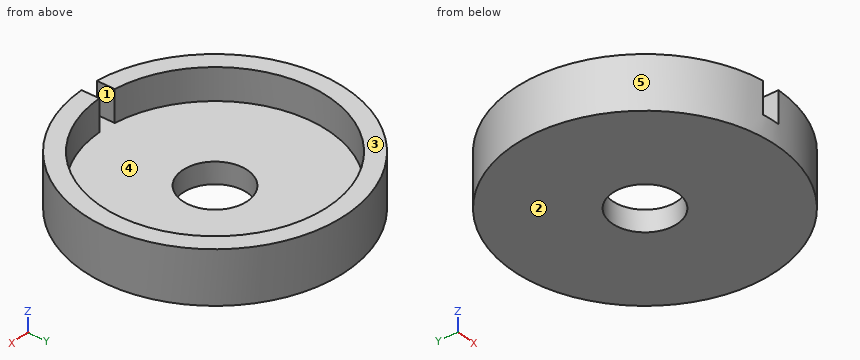
from build123d import *

# Parameters (mm, degrees)
F0_R     = 7.5
F1_DEPTH = 3
F2_R     = 6.5000001341
F3_DEPTH = 1.8
F5_DEPTH = 1.8
F6_R     = 1.85
F7_DEPTH = 2


with BuildPart() as f1:
    # F0 (on Top) → F1 (new body)
    with BuildSketch(Plane.XY):
        Circle(F0_R)
    extrude(amount=F1_DEPTH)

    # F2 (on face) → F3 (cut)
    with BuildSketch(Plane.XY.offset(3)):
        Circle(F2_R)
    extrude(amount=-F3_DEPTH, mode=Mode.SUBTRACT)

    # F4 (on face) → F5 (cut)
    with BuildSketch(Plane.XY.offset(3)):
        with BuildLine():
            Line((0, -7.5), (0, -6.5000001341))
            ThreePointArc((0, -6.5000001341), (-0.4891376474, -6.4815697254), (-0.9755014466, -6.4263830162))
            Line((-0.9755014466, -6.4263830162), (-0.9755014466, -7.4362891907))
            ThreePointArc((-0.9755014466, -7.4362891907), (-0.4887898678, -7.4840553489), (0, -7.5))
        make_face()
    extrude(amount=-F5_DEPTH, mode=Mode.SUBTRACT)

    # F6 (on face) → F7 (cut)
    with BuildSketch(Plane.XY.offset(1.2)):
        Circle(F6_R)
    extrude(amount=-F7_DEPTH, mode=Mode.SUBTRACT)


solid = f1.part
The model under review builds one solid part; all positions refer to its coordinate system, in mm. Face numbers are marked on the shaded views. A direction names the side the tool comes from. Give positions to 0.01 mm unless a question says otherwise; leave off trailing zeros. Loops run counter-clockwise (first coordinate to the right, second up) from the corner with the lowest first, then second, coordinate; pieces in that order, holes last. Notation, with made-up numbers: (85.5, 10.5) -> (143.5, 10.5) arc R15 cw to (143.5, 36.5) -> close; hole circle Ø11 at (-11, 47). An arc over 180 degrees is marked (long way). Write each question's results on one line, items separated by ' | '.
1) Take a section at A-A, the plane z = 1. Give the boundary of the cut face in (x, y).
Conclusion:
outline: circle Ø15 at (0, 0); hole circle Ø3.7 at (0, 0)
2) Take a section at C-C, the plane x = -4.25. Give the boundary of the cut face in (y, z).
Conclusion:
outline: (-6.18, 0) -> (6.18, 0) -> (6.18, 3) -> (4.92, 3) -> (4.92, 1.2) -> (-4.92, 1.2) -> (-4.92, 3) -> (-6.18, 3) -> close
3) Take a section at B-B, the plane y = 1.5. Give the boundary of the cut face in (x, z).
Conclusion:
outline: (-7.35, 0) -> (-1.08, 0) -> (-1.08, 1.2) -> (-6.32, 1.2) -> (-6.32, 3) -> (-7.35, 3) -> close; (1.08, 0) -> (7.35, 0) -> (7.35, 3) -> (6.32, 3) -> (6.32, 1.2) -> (1.08, 1.2) -> close
4) Tool access review of the marked faces 1 and 2: name each direction out of +Z, -Z, +X, -X, +Y, -Y from which nothing blocks a thin tool from reaching the whole face with its end or side.
Conclusion:
face 1: +Z, -Y | face 2: -Z, +X, -X, +Y, -Y
5) For line 1 along X through (y, z) = (0, 1.8); line 2 along Z through (x, y) = (3.75, -0.5); line 3 along Y through (x, z) = (0, 1), list the stretches that pass through material, from the lowest coordinate up. Write a range as from..to.
Conclusion:
line 1: x = -7.5..-6.5, 6.5..7.5 | line 2: z = 0..1.2 | line 3: y = -7.5..-1.85, 1.85..7.5
6) Draft analysis for pull direction X (two halves, no side actions). For the marked faces 3, 4 and 5, state which applies: pulls with the +X half, pulls with the -X half, needs draft (parallel to the pull), parting line crosses it, or undercut.
Conclusion:
face 3: needs draft | face 4: undercut | face 5: parting line crosses it
7) Take a section at D-D, the plane y = -2.25. Give the boundary of the cut face in (x, z).
Conclusion:
outline: (-7.15, 0) -> (7.15, 0) -> (7.15, 3) -> (6.1, 3) -> (6.1, 1.2) -> (-6.1, 1.2) -> (-6.1, 3) -> (-7.15, 3) -> close
8) Insertion check: pin 1 Ø1.1 at (y, z) = (-7, 2) entering from +X; pin 2 Ø0.8 at (y, z) = (-7, 2) entering from -X; pin 3 Ø1 at (x, z) = (4.5, 1.5) entering from +Y. Each pin has a flat end and moves straight along its axis. Give the tip position at first contact, or say it passes through.
Conclusion:
pin 1: stops at x = 3.83 | pin 2: stops at x = -3.56 | pin 3: stops at y = 6.34
